The listing builds one solid part. Answer for the finished solid, in the listing's coordinates (mm). A direction names the side the tool comes from. Round coordinates to 2 decimals unless told otherwise and drop trailing zeros. Order: outer loops, then holes, each group sorted by start corner. A loop starts at its lowest first (then second) coordinate and runs counter-clockwise, first axis right, second up. Notation, with made-up numbers: (73.25, 17) - (128.25, 17) arc R37 cw to (128.25, 53) - close; hole circle Ø11 at (64, 65.25). An arc over 180 degrees is marked (long way). Write item = value, one per line.
from build123d import *

# Parameters (mm, degrees)
BOSS_EXTRUDE1_DEPTH      = 30
SKETCH2_W                = 26.926999998
SKETCH2_H                = 60
BOSS_EXTRUDE2_DEPTH      = 200
BOSS_EXTRUDE3_START      = 30
BOSS_EXTRUDE3_DEPTH      = 30
BOSS_EXTRUDE4_DEPTH      = 4.0365
BOSS_EXTRUDE4_DEPTH_BACK = 30.9635
BOSS_EXTRUDE5_DEPTH      = 10
FILLET1_R                = 30
SKETCH7_W                = 260
SKETCH7_H                = 710
CUT_EXTRUDE1_DEPTH       = 1059.06427026
CHAMFER1_SIZE            = 2
CHAMFER2_SIZE            = 2
CHAMFER3_SIZE            = 2
CHAMFER4_SIZE            = 2
CHAMFER6_SIZE            = 2


with BuildPart() as part:
    # Sketch1 → Boss-Extrude1 (new body)
    with BuildSketch(Plane.XY):
        with BuildLine():
            Line((0, 0), (1500, 0))
            Line((1500, 0), (1500, -100))
            Line((1500, -100), (1465, -100))
            ThreePointArc((1465, -100), (750, -57.245588357), (35, -100))
            Line((35, -100), (0, -100))
            Line((0, -100), (0, 0))
        make_face()
    extrude(amount=BOSS_EXTRUDE1_DEPTH)

    # Sketch2 → Boss-Extrude2 (add)
    with BuildSketch(Plane(origin=(0, 0, 0), x_dir=(-1, 0, 0), z_dir=(0, 0, -1))):
        with Locations((-1482.5, -70)):
            Rectangle(SKETCH2_W, SKETCH2_H)
        with Locations((-17.5, -70)):
            Rectangle(SKETCH2_W, SKETCH2_H)
    extrude(amount=BOSS_EXTRUDE2_DEPTH)

    # Sketch3 → Boss-Extrude3 (add)
    with BuildSketch(Plane(origin=(0, 0, -200), x_dir=(-1, 0, 0), z_dir=(0, 0, -1)).offset(BOSS_EXTRUDE3_START)):
        with BuildLine():
            Line((0, -100), (0, 0))
            Line((0, 0), (-1500, 0))
            Line((-1500, 0), (-1500, -100))
            Line((-1500, -100), (-1465, -100))
            ThreePointArc((-1465, -100), (-750, -57.245588357), (-35, -100))
            Line((-35, -100), (0, -100))
        make_face()
    extrude(amount=-BOSS_EXTRUDE3_DEPTH)

    # Sketch5 → Boss-Extrude4 (add, two sides: drawn at the far end of the back side and taken through both)
    with BuildSketch(Plane.ZY.offset(-4.036500001).offset(-BOSS_EXTRUDE4_DEPTH_BACK)):
        Polygon((-200, -100), (0, -100), (30, -100), (30, -115), (-75, -160), (-25, -700), (-100, -700), (-175, -700), (-125, -160), (-230, -115), (-230, -100), align=None)
    extrude(amount=BOSS_EXTRUDE4_DEPTH + BOSS_EXTRUDE4_DEPTH_BACK)

    # Sketch6 → Boss-Extrude5 (add)
    with BuildSketch(Plane.XZ.offset(700)):
        Polygon((0, -25), (0, 5), (50, 5), (50, -205), (0, -205), (0, -175), align=None)
    extrude(amount=BOSS_EXTRUDE5_DEPTH)

    # Fillet1
    fillet1_edges = [part.edges().sort_by_distance(p)[0] for p in [
        (50, -705, -205),
        (50, -705, 5),
    ]]
    fillet(fillet1_edges, radius=FILLET1_R)

    # Sketch7 → Cut-Extrude1 (cut, through all)
    with BuildSketch(Plane(origin=(750, 0, 0), x_dir=(0, 0, -1), z_dir=(1, 0, 0))):
        with Locations((100, -355)):
            Rectangle(SKETCH7_W, SKETCH7_H)
    extrude(amount=CUT_EXTRUDE1_DEPTH, mode=Mode.SUBTRACT)

    # Mirror2: part across plane


with BuildPart() as part_1:
    add(part.part)
    add(part.part.mirror(Plane(origin=(750, 0, 0), x_dir=(0, 0, 1), z_dir=(1, 0, 0))))

    # Chamfer1
    chamfer1_edges = [part_1.edges().sort_by_distance(p)[0] for p in [
        (750, 0, 30),
        (750, 0, 0),
        (750, 0, -200),
        (750, 0, -230),
    ]]
    chamfer(chamfer1_edges, length=CHAMFER1_SIZE)

    # Chamfer2
    chamfer2_edges = [part_1.edges().sort_by_distance(p)[0] for p in [
        (1495.963499999, -40, -100),
        (1469.036500001, -40, -100),
        (4.036500001, -40, -100),
        (30.963499999, -40, -100),
    ]]
    chamfer(chamfer2_edges, length=CHAMFER2_SIZE)

    # Chamfer3
    chamfer3_edges = [part_1.edges().sort_by_distance(p)[0] for p in [
        (1464.999999999, -107.5, -230),
        (1464.999999999, -137.5, -177.5),
        (1464.999999999, -430, -150),
        (1464.999999999, -430, -50),
        (1464.999999999, -137.5, -22.5),
        (1464.999999999, -107.5, 30),
        (35.000000001, -107.5, 30),
        (35.000000001, -137.5, -22.5),
        (35.000000001, -430, -50),
        (35.000000001, -430, -150),
        (35.000000001, -137.5, -177.5),
        (35.000000001, -107.5, -230),
    ]]
    chamfer(chamfer3_edges, length=CHAMFER3_SIZE)

    # Chamfer4
    chamfer4_edges = [part_1.edges().sort_by_distance(p)[0] for p in [
        (50, -700, -100),
        (10, -700, 5),
        (41.213203436, -700, -3.786796564),
        (41.213203436, -700, -196.213203436),
        (1450, -700, -100),
        (1490, -700, 5),
        (1490, -700, -205),
        (1458.786796564, -700, -196.213203436),
        (1458.786796564, -700, -3.786796564),
        (10, -700, -205),
    ]]
    chamfer(chamfer4_edges, length=CHAMFER4_SIZE)

    # Chamfer6
    # the kernel refuses this chamfer: 2 mm, written as the material it takes off along each edge
    with BuildSketch(Plane(origin=(750, -6057.245588357, 30), x_dir=(0.1203510488799101, 0.9927313962162704, 0), z_dir=(0.9927313962162704, -0.1203510488799101, 0))) as chamfer6_piece_1_section:
        Polygon((6000 + CHAMFER6_SIZE, 0), (6000, -CHAMFER6_SIZE), (6000, 0), align=None)
    chamfer6_piece_1 = revolve(axis=Axis((750, -6057.245588357, 30), (0, 0, 1)), revolution_arc=13.824726066, mode=Mode.PRIVATE)
    chamfer6_piece_1 = split(chamfer6_piece_1, bisect_by=Plane(origin=(1466.125003015, -99.334691053, 29.125003016), z_dir=(-0.7071067811865476, 0, 0.7071067811865476)), keep=Keep.TOP, mode=Mode.PRIVATE)
    chamfer6_piece_1 = split(chamfer6_piece_1, bisect_by=Plane(origin=(749.625001683, -99.334691053, -686.625001682), z_dir=(0.7071067811865476, 0, 0.7071067811865476)), keep=Keep.TOP, mode=Mode.PRIVATE)
    add(chamfer6_piece_1, mode=Mode.SUBTRACT)
    with BuildSketch(Plane(origin=(750, -6057.245588357, -200), x_dir=(-0.12001774996908876, 0.9927717460183672, 0), z_dir=(-0.9927717460183672, -0.12001774996908876, 0))) as chamfer6_piece_2_section:
        Polygon((6000 + CHAMFER6_SIZE, 0), (6000, CHAMFER6_SIZE), (6000, 0), align=None)
    chamfer6_piece_2 = revolve(axis=Axis((750, -6057.245588357, -200), (0, 0, -1)), revolution_arc=13.786253962, mode=Mode.PRIVATE)
    chamfer6_piece_2 = split(chamfer6_piece_2, bisect_by=Plane(origin=(33.165042668, -100, -200.593649662), z_dir=(0, 1, 0)), keep=Keep.TOP, mode=Mode.PRIVATE)
    chamfer6_piece_2 = split(chamfer6_piece_2, bisect_by=Plane(origin=(1469.036500001, -99.402070314, -200.593649662), z_dir=(-1, 0, 0)), keep=Keep.TOP, mode=Mode.PRIVATE)
    chamfer6_piece_2 = split(chamfer6_piece_2, bisect_by=Plane(origin=(30.963499999, -99.402070314, -200.593649662), z_dir=(1, 0, 0)), keep=Keep.TOP, mode=Mode.PRIVATE)
    add(chamfer6_piece_2, mode=Mode.SUBTRACT)
    with BuildSketch(Plane(origin=(750, -6057.245588357, 0), x_dir=(0.12001774996908958, 0.9927717460183672, 0), z_dir=(0.9927717460183672, -0.12001774996908958, 0))) as chamfer6_piece_3_section:
        Polygon((6000 + CHAMFER6_SIZE, 0), (6000, CHAMFER6_SIZE), (6000, 0), align=None)
    chamfer6_piece_3 = revolve(axis=Axis((750, -6057.245588357, 0), (0, 0, 1)), revolution_arc=13.786253962, mode=Mode.PRIVATE)
    chamfer6_piece_3 = split(chamfer6_piece_3, bisect_by=Plane(origin=(1466.834957332, -100, 0.593649662), z_dir=(0, 1, 0)), keep=Keep.TOP, mode=Mode.PRIVATE)
    chamfer6_piece_3 = split(chamfer6_piece_3, bisect_by=Plane(origin=(1469.036500001, -99.402070314, 0.593649662), z_dir=(-1, 0, 0)), keep=Keep.TOP, mode=Mode.PRIVATE)
    chamfer6_piece_3 = split(chamfer6_piece_3, bisect_by=Plane(origin=(30.963499999, -99.402070314, 0.593649662), z_dir=(1, 0, 0)), keep=Keep.TOP, mode=Mode.PRIVATE)
    add(chamfer6_piece_3, mode=Mode.SUBTRACT)
    with BuildSketch(Plane(origin=(750, -6057.245588357, -230), x_dir=(-0.12035104887990915, 0.9927313962162705, 0), z_dir=(-0.9927313962162705, -0.12035104887990915, 0))) as chamfer6_piece_4_section:
        Polygon((6000 + CHAMFER6_SIZE, 0), (6000, -CHAMFER6_SIZE), (6000, 0), align=None)
    chamfer6_piece_4 = revolve(axis=Axis((750, -6057.245588357, -230), (0, 0, -1)), revolution_arc=13.824726066, mode=Mode.PRIVATE)
    chamfer6_piece_4 = split(chamfer6_piece_4, bisect_by=Plane(origin=(750.374998317, -99.334691053, 486.625001682), z_dir=(-0.7071067811865476, 0, -0.7071067811865476)), keep=Keep.TOP, mode=Mode.PRIVATE)
    chamfer6_piece_4 = split(chamfer6_piece_4, bisect_by=Plane(origin=(33.874996985, -99.334691053, -229.125003016), z_dir=(0.7071067811865476, 0, -0.7071067811865476)), keep=Keep.TOP, mode=Mode.PRIVATE)
    add(chamfer6_piece_4, mode=Mode.SUBTRACT)


solid = part_1.part
Q1. Section C-C on y = -588 is taken. Determine the outline of the cut face in (x, z), then the cut area to 3 significant figures.
Model answer:
outline = (0, -164.63) - (33, -164.63) - (35, -162.62) - (35, -37.38) - (33, -35.37) - (0, -35.37) - close; (1465, -162.62) - (1467, -164.63) - (1500, -164.63) - (1500, -35.37) - (1467, -35.37) - (1465, -37.38) - close
area = 9,040 mm^2
Q2. For faces 1 (the face through (4.037, -71, -99)), 2 (the face through (1459.021, -706.056, -3.555)), 3 (the face through (1469.037, -71, -99)), 4 (the face through (16.7, -137.8, -176.8)), determine the directions among +Z, -Z, +X, -X, +Y, -Y from which every point of the face is accessible in a straight line to the end or side of a thin tool.
Model answer:
face_1 = -X, +Y
face_2 = +Z, -Y
face_3 = +Y
face_4 = -Z, +X, -X
Q3. Flat-ended cylindrical pins translate along their axes: P1, Ø6.5, axis at x = 14, y = -707, coming from the -Z side; P2, Ø18.5, axis at x = 14, z = -149, coming from the +Y side; P3, Ø17.5, axis at y = -61, z = -122, coming from the +X side. Find the tip coordinate at first contact, or state that the pin passes through.
Model answer:
P1 = -205
P2 = -40
P3 = 1495.96
Q4. Section A-A on y = -474.5 is taken. Determine the outline of the cut face in (x, z), then the cut area to 3 significant figures.
Model answer:
outline = (0, -154.12) - (33, -154.12) - (35, -152.11) - (35, -47.89) - (33, -45.88) - (0, -45.88) - close; (1465, -152.11) - (1467, -154.12) - (1500, -154.12) - (1500, -45.88) - (1467, -45.88) - (1465, -47.89) - close
area = 7,570 mm^2
Q5. Find the intervals of material crossed by line 1 (X direction, y = -59.5, z = -64); line 2 (X direction, y = -436.5, z = -85); line 3 (Z direction, x = 163.5, y = -50), in increasing order. Write a range as from..to.
Model answer:
line_1 = 4.04..30.96, 1469.04..1495.96
line_2 = 0..35, 1465..1500
line_3 = -230..-200, 0..30
Q6. Section B-B on z = -41 is taken. Count the separate pieces of the cut face and the enclosed holes in it, then the cut area to 3 significant figures.
Model answer:
separate_pieces = 4
enclosed_holes = 0
area = 19,400 mm^2
Q7. Determine the mould class of faces 5 (the face through (1459.021, -706.056, -196.445)), 6 (the face through (1483.27, -433.78, -150.35)), 7 (the face through (1495.963, -71, -99)) for opening direction X: released by +X, released by -X, zero draft, split by the parting line, or undercut.
Model answer:
face_5 = undercut
face_6 = zero draft
face_7 = released by +X
